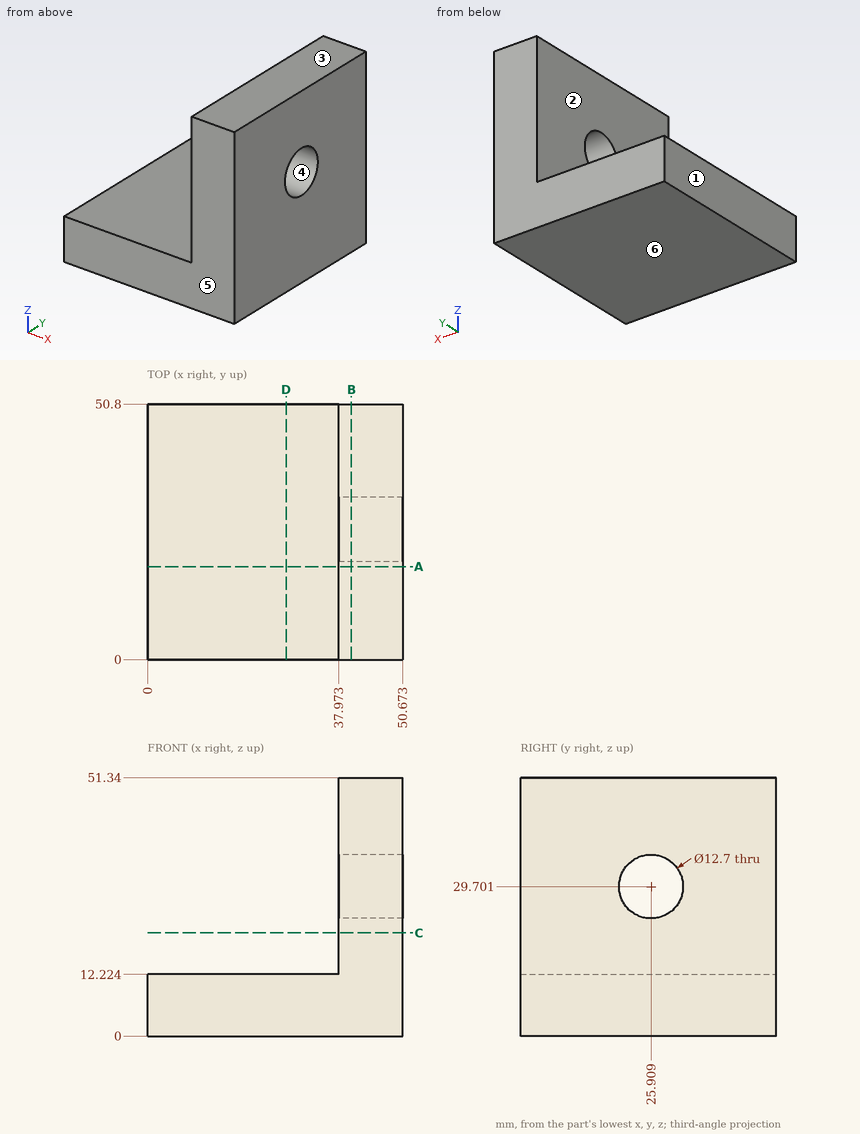
Could you check a few things on this drawing? It's one solid part, dimensions in mm from its lowest x, y, z. A direction names the side the tool comes from. Give positions to 0.01 mm unless a question says otherwise; leave off trailing zeros. Order: outer loops, then holes, each group sorted by start corner. A loop starts at its lowest first (then second) coordinate and runs counter-clockwise, first axis right, second up. Notation, with made-up numbers: (63, -25.75) - (91, -25.75) arc R18 cw to (91, -20.75) - close; hole circle Ø4 at (61, -18). An arc over 180 degrees is marked (long way). Answer as a JSON object with one key per item and string values. Group by question number.
Item 1: If we section it at D-D on x = 27.5: Please give me the cut outline in (y, z).
Item 2: If we section it at A-A on y = 18.5: Please give me the cut outline in (x, z).
Item 3: If we section it at C-C on z = 20.5: Please give me the cut outline in (x, y), and give its area (3 significant figures).
Item 4: If we mould it in two halves opening along Z, with no side actions, what happens to the marked faces 3, 4, 5 and 6? For each: pulls with the +Z half, pulls with the -Z half, needs draft (parallel to the pull), parting line crosses it, or undercut.
Item 5: For P1, Ø8, axis at x = 18, z = 19.5, coming from the -Y side; P2, Ø11.5, axis at y = 30, z = 27, coming from the -X side; P3, Ø2, axis at x = 25.5, y = 35.5, coming from the +Z side, each with a flat end and sliding along its axis, tell me the tip position at first contact or that it passes through.
Item 6: Please list where these lines run through material, in increasing order: probe 1 along Z at (x, y) = (11, 9); probe 2 along X at (y, z) = (4.5, 28.5); probe 3 along Y at (x, z) = (44, 28) (1 decimal).
Item 7: If we section it at B-B on x = 40.5: Please give me the cut outline in (y, z), and give its area (3 significant figures).
Item 8: Which directions (+Z, -Z, +X, -X, +Y, -Y) give clear straight access to the entire face, cutting with the end or side of a thin tool? Please do the marked faces 1 and 2.
Result set:
{
 "1": {"outline": "(0, 0) - (50.8, 0) - (50.8, 12.22) - (0, 12.22) - close"},
 "2": {"outline": "(0, 0) - (50.67, 0) - (50.67, 51.34) - (37.97, 51.34) - (37.97, 12.22) - (0, 12.22) - close"},
 "3": {"outline": "(37.97, 0) - (50.67, 0) - (50.67, 50.8) - (37.97, 50.8) - close", "area": "645 mm²"},
 "4": {"face 3": "pulls with the +Z half", "face 4": "undercut", "face 5": "needs draft", "face 6": "pulls with the -Z half"},
 "5": {"P1": "through", "P2": "x = 37.97", "P3": "z = 12.22"},
 "6": {"probe 1": "0 to 12.22", "probe 2": "37.97 to 50.67", "probe 3": "0 to 19.8, 32 to 50.8"},
 "7": {"outline": "(0, 0) - (50.8, 0) - (50.8, 51.34) - (0, 51.34) - close; hole circle Ø12.7 at (25.91, 29.7)", "area": "2,480 mm²"},
 "8": {"face 1": "+Z, -Z, -X, +Y, -Y", "face 2": "+Z, -X, +Y, -Y"}
}
